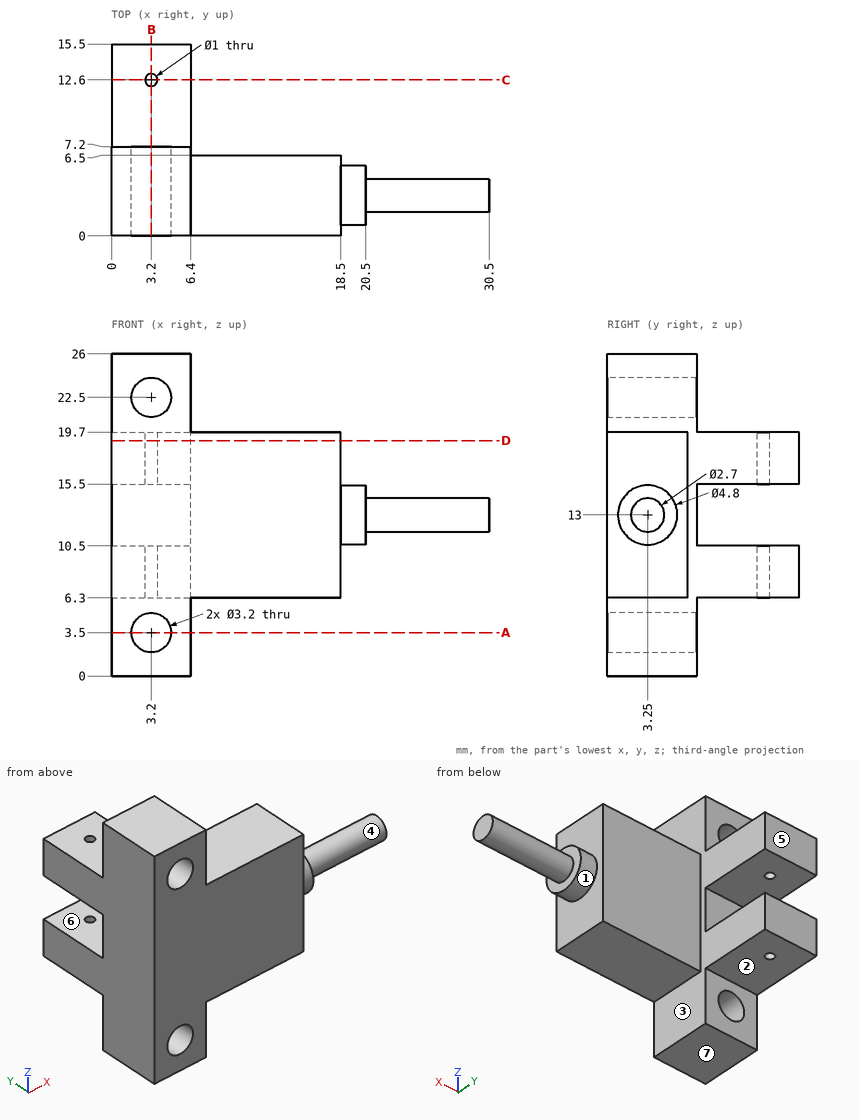
Geometry check sheet. Reference: drawing and pictorial views, mm from the part's lowest x, y, z. A direction names the side the tool comes from. Give positions to 0.01 mm unless a question says otherwise; leave off trailing zeros. Write each loop counter-clockwise with the first axis right and the second up, starting at its lowest first coordinate (ties: lowest second). Pieces come first, ordered by that corner, then holes. Notation, with made-up numbers: M 63.5,3.5 L 98.5,3.5 A12 ccw 98.5,14.5 Z; hole C 83.25,39 d9. An arc over 180 degrees is marked long. Put each result on its own line as item: value. Start each with the question number.
1. Section check C-C (y = 12.6). Record the cut outline in (x, z).
2. Section check D-D (z = 19). Record the cut outline in (x, y).
3. Go/stop test with flat-tipped pins: pin 1 Ø7 at (x, y) = (9.5, 4) entering from +Z; pin 2 Ø4 at (y, z) = (4, 22) entering from +X; pin 3 Ø3 at (x, z) = (3.2, 3.5) entering from -Y; pin 4 Ø4 at (x, z) = (3.2, 22.5) entering from +Y. Record where each tip stops, or that it passes through.
4. Section check B-B (x = 3.2). Record the cut outline in (y, z), and give its area (3 significant figures).
5. Draft check along Z on the marked faces 4, 5, 6 and 7. Enter one of: +Z half, -Z half, draft (parallel to the pull), parting line (faces both ways), or undercut.
6. Scan lines: line 1 along Z through (x, y) = (4.5, 3); line 2 along Y through (x, z) = (3.2, 18.7); line 3 along Y through (x, z) = (2.5, 24.5). Record each from-to range of solid material in increasing order. Write a range as [from, to].
7. Set-up check for the marked faces 1, 2 and 3: record each of +Z, -Z, +X, -X, +Y, -Y from which the full face is reachable in a straight line by a thin tool's end or side.
8. Section check A-A (z = 3.5). Record the cut outline in (x, y), and give its area (3 significant figures).
Answer list:
1. outline: M 0,6.3 L 2.7,6.3 L 2.7,10.5 L 0,10.5 Z; M 0,15.5 L 2.7,15.5 L 2.7,19.7 L 0,19.7 Z; M 3.7,6.3 L 6.4,6.3 L 6.4,10.5 L 3.7,10.5 Z; M 3.7,15.5 L 6.4,15.5 L 6.4,19.7 L 3.7,19.7 Z
2. outline: M 0,0 L 18.5,0 L 18.5,6.5 L 6.4,6.5 L 6.4,15.5 L 0,15.5 Z; hole C 3.2,12.6 d1
3. pin 1: z = 26
3. pin 2: x = 6.4
3. pin 3: through
3. pin 4: y = 7.2
4. outline: M 0,0 L 7.2,0 L 7.2,1.9 L 0,1.9 Z; M 0,5.1 L 7.2,5.1 L 7.2,6.3 L 12.1,6.3 L 12.1,10.5 L 7.2,10.5 L 7.2,15.5 L 12.1,15.5 L 12.1,19.7 L 7.2,19.7 L 7.2,20.9 L 0,20.9 Z; M 0,24.1 L 7.2,24.1 L 7.2,26 L 0,26 Z; M 13.1,6.3 L 15.5,6.3 L 15.5,10.5 L 13.1,10.5 Z; M 13.1,15.5 L 15.5,15.5 L 15.5,19.7 L 13.1,19.7 Z
4. area: 202 mm2
5. face 4: parting line
5. face 5: draft
5. face 6: undercut
5. face 7: -Z half
6. line 1: [0, 2.57], [4.43, 21.57], [23.43, 26]
6. line 2: [0, 12.1], [13.1, 15.5]
6. line 3: [0, 7.2]
7. face 1: +X
7. face 2: -Z, +X, -X, +Y
7. face 3: +X, +Y
8. outline: M 0,0 L 1.6,0 L 1.6,7.2 L 0,7.2 Z; M 4.8,0 L 6.4,0 L 6.4,7.2 L 4.8,7.2 Z
8. area: 23.0 mm2
